Build history of the part. All positions in model axes, mm. Round coordinates to 2 decimals unless told otherwise and drop trailing zeros. Loops run counter-clockwise (first coordinate to the right, second up) from the corner with the lowest first, then second, coordinate; pieces in that order, holes last. Notation, with made-up numbers: M 79.25,-35.75 L 122.25,-35.75 A13 ccw 122.25,-19.75 Z; hole C 21.25,79.5 d7. An arc over 180 degrees is marked long. One line per item, written item: value.
Autodesk Inventor part; units mm, degrees
ref_plane "YZ Plane" through (0, 0, 0) normal (1, 0, 0) x (0, 1, 0)
ref_plane "XZ Plane" through (0, 0, 0) normal (0, 1, 0) x (-1, 0, 0)
ref_plane "XY Plane" through (0, 0, 0) normal (0, 0, 1) x (1, 0, 0)
sketch "Sketch1" plane through (0, 0, 0) normal (1, 0, 0) x (0, 1, 0)
  line L0 (0, -332) -> (-46, -332) construction
  line L1 (-46, -332) -> (-46, -297.4128)
  line L2 (-46, -332) -> (-46, -348.8838)
  line L3 (-85.3886, -374.4631) -> (-125.3109, -356.6885)
  line L4 (-141.9223, -331.1092) -> (-141.9223, -275.0602)
  arc A0 (-85.3886, -374.4631) -> (-46, -348.8838) centre (-74, -348.8838) ccw
  arc A1 (-100.2431, -250.629) -> (-141.9223, -275.0602) centre (-113.9223, -275.0602) ccw
  arc A2 (-46, -297.4128) -> (-60.3209, -272.9817) centre (-74, -297.4128) ccw
  arc A3 (-141.9223, -331.1092) -> (-125.3109, -356.6885) centre (-113.9223, -331.1092) ccw
  line L5 (0, -332) -> (-46, -332) construction
  line L6 (-46, -332) -> (-46, -297.4128)
  line L7 (-46, -332) -> (-46, -348.8838)
  line L8 (-85.3886, -374.4631) -> (-125.3109, -356.6885)
  line L9 (-141.9223, -331.1092) -> (-141.9223, -275.0602)
  arc A4 (-85.3886, -374.4631) -> (-46, -348.8838) centre (-74, -348.8838) ccw
  arc A5 (-100.2431, -250.629) -> (-141.9223, -275.0602) centre (-113.9223, -275.0602) ccw
  arc A6 (-46, -297.4128) -> (-60.3209, -272.9817) centre (-74, -297.4128) ccw
  arc A7 (-141.9223, -331.1092) -> (-125.3109, -356.6885) centre (-113.9223, -331.1092) ccw
  line L10 (0, -332) -> (-46, -332) construction
  line L11 (-46, -332) -> (-46, -297.4128)
  line L12 (-46, -332) -> (-46, -348.8838)
  line L13 (-85.3886, -374.4631) -> (-125.3109, -356.6885)
  line L14 (-141.9223, -331.1092) -> (-141.9223, -275.0602)
  line L15 (-60.3209, -272.9817) -> (-100.2431, -250.629)
  arc A8 (-85.3886, -374.4631) -> (-46, -348.8838) centre (-74, -348.8838) ccw
  arc A9 (-100.2431, -250.629) -> (-141.9223, -275.0602) centre (-113.9223, -275.0602) ccw
  arc A10 (-46, -297.4128) -> (-60.3209, -272.9817) centre (-74, -297.4128) ccw
  arc A11 (-141.9223, -331.1092) -> (-125.3109, -356.6885) centre (-113.9223, -331.1092) ccw
  line L16 (-141.8223, -275.0602) -> (-141.8223, -331.1092)
  arc A12 (-141.8223, -331.1092) -> (-125.2702, -356.5972) centre (-113.9223, -331.1092) ccw
  line L17 (-125.2702, -356.5972) -> (-85.348, -374.3717)
  arc A13 (-85.348, -374.3717) -> (-46.1, -348.8838) centre (-74, -348.8838) ccw
  line L18 (-46.1, -348.8838) -> (-46.1, -332)
  line L19 (-46.1, -332) -> (-46.1, -297.4128)
  arc A14 (-46.1, -297.4128) -> (-60.3697, -273.0689) centre (-74, -297.4128) ccw
  line L20 (-60.3697, -273.0689) -> (-100.292, -250.7163)
  arc A15 (-100.292, -250.7163) -> (-141.8223, -275.0602) centre (-113.9223, -275.0602) ccw
  point P0 (0, 0)
  point P1 (-46, -281)
  point P2 (-46, -392)
  point P3 (-141.9223, -349.2927)
  point P4 (-141.9223, -227.2927)
  point P5 (-46, -281)
  point P6 (-46, -392)
  point P7 (-141.9223, -349.2927)
  point P8 (-141.9223, -227.2927)
  point P9 (-46, -281)
  point P10 (-46, -392)
  point P11 (-141.9223, -349.2927)
  point P12 (-141.9223, -227.2927)
  dimension "d43" = 0
  dimension "d0" = 46
  dimension "d1" = 51
  dimension "d2" = 60
  dimension "d3" = 105
  dimension "d4" = 66
  dimension "d5" = 122
  dimension "d6" = 28
  dimension "d7" = 28
  dimension "d8" = 28
  dimension "d9" = 46
  dimension "d11" = 60
  dimension "d12" = 105
  dimension "d13" = 66
  dimension "d14" = 122
  dimension "d15" = 28
  dimension "d16" = 28
  dimension "d17" = 28
  dimension "d18" = 46
  dimension "d21" = 105
  dimension "d22" = 66
  dimension "d23" = 122
  dimension "d24" = 28
  dimension "d25" = 28
  dimension "d26" = 28
  dimension "d27" = 0.1
extrude "Extrusion1" add sketch "Sketch1" along normal blind 3 contours A15 L20 A14 L19 L18 A13 L17 A12 L16
sketch "Sketch2" plane through (3, 0, 0) normal (1, 0, 0) x (0, 0, -1)
  arc A0 (250.7163, -100.292) -> (275.0602, -141.8223) centre (275.0602, -113.9223) ccw
  arc A1 (374.3717, -85.348) -> (348.8838, -46.1) centre (348.8838, -74) ccw
  arc A2 (297.4128, -46.1) -> (273.0689, -60.3697) centre (297.4128, -74) ccw
  arc A3 (331.1092, -141.8223) -> (356.5972, -125.2702) centre (331.1092, -113.9223) ccw
  circle A4 centre (328.9681, -50.7353) radius 0.5
  line L0 (273.0689, -60.3697) -> (250.7163, -100.292)
  circle A5 centre (264.0532, -86.152) radius 0.5
  line L1 (356.5972, -125.2702) -> (374.3717, -85.348)
  circle A6 centre (360.8666, -103.7379) radius 0.5
  line L2 (275.0602, -141.8223) -> (331.1092, -141.8223)
  circle A7 centre (296.9895, -137.1327) radius 0.5
  point P0 (0, 0)
extrude "Extrusion2" cut sketch "Sketch2" against normal blind 5
chamfer "Chamfer1" distance 0.5 angle 45 1 edges at (3, -86.152, -263.5532)
chamfer "Chamfer2" distance 0.5 angle 45 3 edges at (3, -137.1327, -296.4895) (3, -103.7379, -360.3666) (3, -50.7353, -328.4681)
properties part number "tampa traseira do corpo" material "PET Plastic"
Item 1: Slice it at B-B, the plane z = -365.5. Give the cut face in (x, y).
Check values:
outline: M 0,-105.27 L 3,-105.27 L 3,-51.59 L 0,-51.59 Z
Item 2: Slice it at A-A, the plane y = -97. Give the cut face in (x, z), and give its area (3 significant figures).
Check values:
outline: M 0,-369.18 L 3,-369.18 L 3,-252.56 L 0,-252.56 Z
area: 350 mm2
Item 3: Wall check: line 1 along Y through (x, z) = (0.7, -331.5); line 2 along Y through (x, z) = (0.3, -361); line 3 along Z through (x, y) = (2.15, -113.5). Give the ranges that are in metal, low to high.
Check values:
line 1: y = -141.82 to -46.1
line 2: y = -115.38 to -104.22, -103.26 to -48.87
line 3: z = -361.84 to -247.16
